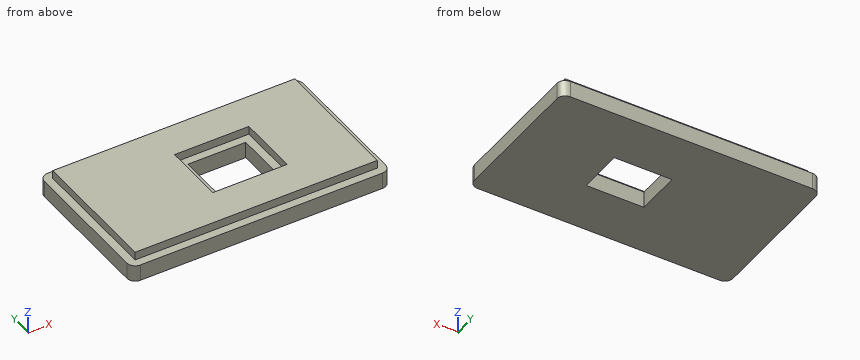
```python
from build123d import *

# Parameters (mm, degrees)
F0_W        = 58.6601923168
F0_H        = 32.2631057742
F0_W_2      = 18
F0_H_2      = 15
F1_DEPTH    = 2
F2_T        = 2
F3_T1_DEPTH = 2
F3_T3_DEPTH = 14
F4_DEPTH    = 4


# Not quite as in the source:
# - a fillet or chamfer that OpenCascade refuses, or shapes differently, is made with other operations: its cross-section is extruded or revolved along the edge and cut away or added
# - a feature names something its author has since deleted; it is built from what else it names


with BuildPart() as f1:
    # F0 (on Top) → F1 (new body)
    with BuildSketch(Plane.XY):
        with Locations((-3.8516821679, 0)):
            Rectangle(F0_W, F0_H)
        Rectangle(F0_W_2, F0_H_2, mode=Mode.SUBTRACT)
    extrude(amount=F1_DEPTH)

    # F2
    f2_openings = [f1.faces().sort_by_distance(p)[0] for p in [
        (24.808942, 0, 2),
    ]]
    offset(amount=F2_T, openings=f2_openings, kind=Kind.INTERSECTION)

    # F3: fillet of radius 2 on 8 edges, made by hand

    # F3_s2 → F3_t1 (join)
    with BuildSketch(Plane.XY):
        with BuildLine():
            ThreePointArc((-31.1817783263, 16.1315528871), (-32.5959918887, 15.5457664495), (-33.1817783263, 14.1315528871))
            Line((-33.1817783263, 14.1315528871), (-33.1817783263, 16.1315528871))
            Line((-33.1817783263, 16.1315528871), (-31.1817783263, 16.1315528871))
        make_face()
        with BuildLine():
            ThreePointArc((-33.1817783263, -14.1315528871), (-32.5959918887, -15.5457664495), (-31.1817783263, -16.1315528871))
            Line((-31.1817783263, -16.1315528871), (-33.1817783263, -16.1315528871))
            Line((-33.1817783263, -16.1315528871), (-33.1817783263, -14.1315528871))
        make_face()
        with BuildLine():
            ThreePointArc((25.4784139905, -14.1315528871), (24.8926275528, -15.5457664495), (23.4784139905, -16.1315528871))
            Line((23.4784139905, -16.1315528871), (25.4784139905, -16.1315528871))
            Line((25.4784139905, -16.1315528871), (25.4784139905, -14.1315528871))
        make_face()
        with BuildLine():
            ThreePointArc((25.4784139905, 14.1315528871), (24.8926275528, 15.5457664495), (23.4784139905, 16.1315528871))
            Line((23.4784139905, 16.1315528871), (25.4784139905, 16.1315528871))
            Line((25.4784139905, 16.1315528871), (25.4784139905, 14.1315528871))
        make_face()
    extrude(amount=F3_T1_DEPTH)

    # F3_s4 → F3_t3 (cut)
    with BuildSketch(Plane.XY.offset(-7)):
        with BuildLine():
            ThreePointArc((25.4784139905, -18.1315528871), (26.8926275528, -17.5457664495), (27.4784139905, -16.1315528871))
            Line((27.4784139905, -16.1315528871), (27.4784139905, -18.1315528871))
            Line((27.4784139905, -18.1315528871), (25.4784139905, -18.1315528871))
        make_face()
        with BuildLine():
            ThreePointArc((27.4784139905, 16.1315528871), (26.8926275528, 17.5457664495), (25.4784139905, 18.1315528871))
            Line((25.4784139905, 18.1315528871), (27.4784139905, 18.1315528871))
            Line((27.4784139905, 18.1315528871), (27.4784139905, 16.1315528871))
        make_face()
        with BuildLine():
            ThreePointArc((-35.1817783263, 16.1315528871), (-34.5959918887, 17.5457664495), (-33.1817783263, 18.1315528871))
            Line((-33.1817783263, 18.1315528871), (-35.1817783263, 18.1315528871))
            Line((-35.1817783263, 18.1315528871), (-35.1817783263, 16.1315528871))
        make_face()
        with BuildLine():
            ThreePointArc((-35.1817783263, -16.1315528871), (-34.5959918887, -17.5457664495), (-33.1817783263, -18.1315528871))
            Line((-33.1817783263, -18.1315528871), (-35.1817783263, -18.1315528871))
            Line((-35.1817783263, -18.1315528871), (-35.1817783263, -16.1315528871))
        make_face()
    extrude(amount=F3_T3_DEPTH, mode=Mode.SUBTRACT)

    # F0 (on Top) → F4 (join)
    with BuildSketch(Plane.XY):
        with Locations((-3.8516821679, 0)):
            Rectangle(F0_W, F0_H)
        Rectangle(F0_W_2, F0_H_2, mode=Mode.SUBTRACT)
    extrude(amount=F4_DEPTH)


solid = f1.part
```
The listing builds one solid part. Answer for the finished solid, in the listing's coordinates (mm). Give positions to 0.01 mm unless a question says otherwise; leave off trailing zeros. Loops run counter-clockwise (first coordinate to the right, second up) from the corner with the lowest first, then second, coordinate; pieces in that order, holes last. Notation, with made-up numbers: (57, 37) - (66, 37) arc R17 cw to (66, 46) - close; hole circle Ø10 at (68, -14.5). An arc over 180 degrees is marked (long way). Answer as CSV lines item,"result". Start each with the question number.
Item 1: A cutting plane is placed at B-B on x = -4. Determine the outline of the cut face in (y, z), then the cut area to 3 significant figures.
Item 2: A cutting plane is placed at C-C on z = 0.6. Determine the outline of the cut face in (x, y).
Item 3: Each of these flat-tipped pins is pushed along its axis until it touches: pin 1 (1.6 mm diameter, centred on y = 1, z = 3, fed in from +X); pin 2 (2 mm diameter, centred on x = -3.5, z = 3.5, fed in from -Y); pin 3 (1.6 mm diameter, centred on x = -2.5, z = 3, fed in from +Y). Where does it stop, or does it pass through?
Item 4: Find the intervals of material crossed by line 1 (X direction, y = 7, z = 2.2); line 2 (Y direction, x = 5, z = 0.1); line 3 (X direction, y = 2.5, z = -1.35), in increasing order. Write a range as from..to.
Item 5: A cutting plane is placed at D-D on x = -12.5. Determine the outline of the cut face in (y, z), then the cut area to 3 significant figures.
Item 6: A cutting plane is placed at A-A on y = 2. Determine the outline of the cut face in (x, z).
Found:
1,outline,"(-18.13, -2) - (-5.5, -2) - (-5.5, 2) - (-7.5, 2) - (-7.5, 4) - (-16.13, 4) - (-16.13, 2) - (-18.13, 2) - close; (5.5, -2) - (18.13, -2) - (18.13, 2) - (16.13, 2) - (16.13, 4) - (7.5, 4) - (7.5, 2) - (5.5, 2) - close"
1,area,"136 mm^2"
2,outline,"(-35.18, -16.13) arc R2 ccw to (-33.18, -18.13) - (25.48, -18.13) arc R2 ccw to (27.48, -16.13) - (27.48, 16.13) arc R2 ccw to (25.48, 18.13) - (-33.18, 18.13) arc R2 ccw to (-35.18, 16.13) - close; hole (-7, -5.5) - (7, -5.5) - (7, 5.5) - (-7, 5.5) - close"
3,pin 1,"stops at x = 25.48"
3,pin 2,"stops at y = -16.13"
3,pin 3,"stops at y = 16.13"
4,line 1,"x = -33.18..-9, 9..25.48"
4,line 2,"y = -18.13..-5.5, 5.5..18.13"
4,line 3,"x = -35.18..-7, 7..27.48"
5,outline,"(-18.13, -2) - (18.13, -2) - (18.13, 2) - (16.13, 2) - (16.13, 4) - (-16.13, 4) - (-16.13, 2) - (-18.13, 2) - close"
5,area,"210 mm^2"
6,outline,"(-35.18, -2) - (-7, -2) - (-7, 2) - (-9, 2) - (-9, 4) - (-33.18, 4) - (-33.18, 2) - (-35.18, 2) - close; (7, -2) - (27.48, -2) - (27.48, 2) - (25.48, 2) - (25.48, 4) - (9, 4) - (9, 2) - (7, 2) - close"
